from build123d import *

# Parameters (mm, degrees)
BOSS_EXTRUDE1_DEPTH = 70
CUT_EXTRUDE3_DEPTH  = 70
SKETCH3_R           = 2.75
CUT_EXTRUDE6_DEPTH  = 5


with BuildPart() as part:
    # Sketch1 → Boss-Extrude1 (new body)
    with BuildSketch(Plane(origin=(0, 0, 0), x_dir=(1, 0, 0), z_dir=(0, 1, 0))):
        with BuildLine():
            Line((15.254575611, 35.990242765), (15.254575611, 44.990242765))
            ThreePointArc((15.254575611, 44.990242765), (13.790109517, 48.525776671), (10.254575611, 49.990242765))
            Line((10.254575611, 49.990242765), (-50.745424389, 49.990242765))
            ThreePointArc((-50.745424389, 49.990242765), (-99.757685432, 0), (-50.745424389, -49.990242765))
            Line((-50.745424389, -49.990242765), (10.254575611, -49.990242765))
            ThreePointArc((10.254575611, -49.990242765), (13.790109517, -48.525776671), (15.254575611, -44.990242765))
            Line((15.254575611, -44.990242765), (15.254575611, -35.990242765))
            ThreePointArc((15.254575611, -35.990242765), (16.133255268, -33.868922422), (18.254575611, -32.990242765))
            Line((18.254575611, -32.990242765), (22.711934924, -32.990242765))
            ThreePointArc((22.711934924, -32.990242765), (23.859985221, -33.218604168), (24.833255268, -33.868922422))
            Line((24.833255268, -33.868922422), (40.954575611, -49.990242765))
            Line((40.954575611, -49.990242765), (50.745424389, -49.990242765))
            Line((50.745424389, -49.990242765), (94.067824265, -49.990242765))
            ThreePointArc((94.067824265, -49.990242765), (96.567824265, -50.660115747), (98.397951284, -52.490242765))
            Line((98.397951284, -52.490242765), (114.280717029, -80))
            Line((114.280717029, -80), (134.280717029, -80))
            Line((134.280717029, -80), (134.280717029, 80))
            Line((134.280717029, 80), (114.280717029, 80))
            Line((114.280717029, 80), (98.397951284, 52.490242765))
            ThreePointArc((98.397951284, 52.490242765), (96.567824265, 50.660115747), (94.067824265, 49.990242765))
            Line((94.067824265, 49.990242765), (50.745424389, 49.990242765))
            Line((50.745424389, 49.990242765), (40.954575611, 49.990242765))
            Line((40.954575611, 49.990242765), (24.833255268, 33.868922422))
            ThreePointArc((24.833255268, 33.868922422), (23.859985221, 33.218604168), (22.711934924, 32.990242765))
            Line((22.711934924, 32.990242765), (18.254575611, 32.990242765))
            ThreePointArc((18.254575611, 32.990242765), (16.133255268, 33.868922422), (15.254575611, 35.990242765))
        make_face()
    extrude(amount=BOSS_EXTRUDE1_DEPTH)

    # Sketch5 → Cut-Extrude3 (cut)
    with BuildSketch(Plane(origin=(0, 70, 0), x_dir=(1, 0, 0), z_dir=(0, 1, 0))):
        with BuildLine():
            Line((116.012767836, 77), (100.996027496, 50.990242765))
            ThreePointArc((100.996027496, 50.990242765), (98.067824265, 48.062039535), (94.067824265, 46.990242765))
            Line((94.067824265, 46.990242765), (42.197216298, 46.990242765))
            Line((42.197216298, 46.990242765), (26.954575611, 31.747602078))
            ThreePointArc((26.954575611, 31.747602078), (25.008035518, 30.44696557), (22.711934924, 29.990242765))
            Line((22.711934924, 29.990242765), (18.254575611, 29.990242765))
            ThreePointArc((18.254575611, 29.990242765), (14.011934924, 31.747602078), (12.254575611, 35.990242765))
            Line((12.254575611, 35.990242765), (12.254575611, 44.990242765))
            ThreePointArc((12.254575611, 44.990242765), (11.668789174, 46.404456328), (10.254575611, 46.990242765))
            Line((10.254575611, 46.990242765), (-50.715330899, 46.990242765))
            ThreePointArc((-50.715330899, 46.990242765), (-96.757685432, 0), (-50.715330899, -46.990242765))
            Line((-50.715330899, -46.990242765), (10.254575611, -46.990242765))
            ThreePointArc((10.254575611, -46.990242765), (11.668789174, -46.404456328), (12.254575611, -44.990242765))
            Line((12.254575611, -44.990242765), (12.254575611, -35.990242765))
            ThreePointArc((12.254575611, -35.990242765), (14.011934924, -31.747602078), (18.254575611, -29.990242765))
            Line((18.254575611, -29.990242765), (22.711934924, -29.990242765))
            ThreePointArc((22.711934924, -29.990242765), (25.008035518, -30.44696557), (26.954575611, -31.747602078))
            Line((26.954575611, -31.747602078), (42.197216298, -46.990242765))
            Line((42.197216298, -46.990242765), (94.067824265, -46.990242765))
            ThreePointArc((94.067824265, -46.990242765), (98.067824265, -48.062039535), (100.996027496, -50.990242765))
            Line((100.996027496, -50.990242765), (116.012767836, -77))
            Line((116.012767836, -77), (131.280717029, -77))
            Line((131.280717029, -77), (131.280717029, 77))
            Line((131.280717029, 77), (116.012767836, 77))
        make_face()
    extrude(amount=-CUT_EXTRUDE3_DEPTH, mode=Mode.SUBTRACT)

    # Sketch3 → Cut-Extrude6 (cut)
    with BuildSketch(Plane(origin=(134.280717029, 0, 0), x_dir=(0, 0, -1), z_dir=(1, 0, 0))):
        with Locations((-74.64699859, 15)):
            Circle(SKETCH3_R)
        with Locations((-74.64699859, 35)):
            Circle(SKETCH3_R)
        with Locations((74.64699859, 35)):
            Circle(SKETCH3_R)
        with Locations((74.64699859, 15)):
            Circle(SKETCH3_R)
    extrude(amount=-CUT_EXTRUDE6_DEPTH, mode=Mode.SUBTRACT)


solid = part.part
Design review of the part built by this model. Coordinates are the model's own, in mm. A direction names the side the tool comes from. Coordinates: 2 decimals unless noted, no trailing zeros. Loops run counter-clockwise (first coordinate to the right, second up) from the corner with the lowest first, then second, coordinate; pieces in that order, holes last. Notation, with made-up numbers: (82.25, 39.5) - (98.25, 39.5) arc R20 cw to (98.25, 76.5) - close; hole circle Ø11 at (-11.5, -3). An arc over 180 degrees is marked (long way). Use CSV: the item, a comma, the result in double quotes. Start each with the question number.
1. Clearance check with flat-ended pins moving along their axes: pin 1 (1.3 mm diameter, centred on x = 20.5, y = 35.5, fed in from -Z); pin 2 (15.5 mm diameter, centred on x = 78.5, y = 34, fed in from +Z); pin 3 (9 mm diameter, centred on y = 35, z = 74.65, fed in from +X); pin 4 (4.5 mm diameter, centred on y = 45, z = 39.5, fed in from -X). State where each tip first meets the part, or that it passes through.
2. To check wall thickness, follow probe 1 along Z at (x, y) = (133.2, 35); probe 2 along Z at (x, y) = (65, 49); probe 3 along Z at (x, y) = (130, 35). State the ranges of each line that lie inside material, in increasing order.
3. Add section B-B on x = -13. Give the boundary of the cut face in (y, z), plus the area to 3 significant figures.
4. Mouldability with a two-part tool opening along Z and no side actions: class faces 5 (the flat face through (34.683, 35.49, -39.476)), 6 (the flat face through (-21, 35, 49.99)), 7 (the flat face through (124, 35, -80)) as released by +Z, released by -Z, zero draft, split by the parting line, or undercut.
5. Add section A-A on z = 0. Give the boundary of the cut face in (x, y), plus the area to 3 significant figures.
6. For faces 1 (the flat face through (68, 35, -49.99)), 2 (the cylindrical face through (132.927, 15.121, 77.394)), 3 (the cylindrical face through (13.751, 34.51, 48.564)), 4 (the cylindrical face through (14.06, 35.49, -31.7)), list the 3-axis set-ups (+Z, -Z, +X, -X, +Y, -Y) from which the entire face can be reached by the end or side of a thin tool; tool diameter is ignored.
Resolved:
1,pin 1,"z = -32.99"
1,pin 2,"z = 49.99"
1,pin 3,"x = 134.28"
1,pin 4,"x = -83.11"
2,probe 1,"-80 to -77.4, -71.9 to 71.9, 77.4 to 80"
2,probe 2,"-49.99 to -46.99, 46.99 to 49.99"
2,probe 3,"-80 to -77.4, 77.4 to 80"
3,outline,"(0, -49.99) - (70, -49.99) - (70, -46.99) - (0, -46.99) - close; (0, 46.99) - (70, 46.99) - (70, 49.99) - (0, 49.99) - close"
3,area,"420 mm2"
4,face 5,"undercut"
4,face 6,"released by +Z"
4,face 7,"released by -Z"
5,outline,"(-99.76, 0) - (-96.76, 0) - (-96.76, 70) - (-99.76, 70) - close; (131.28, 0) - (134.28, 0) - (134.28, 70) - (131.28, 70) - close"
5,area,"420 mm2"
6,face 1,"-Z, -X, +Y, -Y"
6,face 2,"+X"
6,face 3,"+Z, +Y, -Y"
6,face 4,"+Y, -Y"
